Autodesk Inventor part; units mm, degrees
ref_plane "YZ Plane" through (0, 0, 0) normal (1, 0, 0) x (0, 1, 0)
ref_plane "XZ Plane" through (0, 0, 0) normal (0, 1, 0) x (-1, 0, 0)
ref_plane "XY Plane" through (0, 0, 0) normal (0, 0, 1) x (1, 0, 0)
sketch "Sketch1" plane through (0, 0, 0) normal (0, 0, 1) x (1, 0, 0)
  circle A0 centre (0, 0) radius 3
  circle A1 centre (0, 0) radius 6
  dimension "d0" = 6
  dimension "d1" = 12
extrude "Extrusion1" add sketch "Sketch1" against normal blind 3
sketch "Sketch2" plane through (0, 0, -3) normal (0, 0, -1) x (-1, 0, 0)
  circle A0 centre (0, 0) radius 7
  circle A1 centre (0, 0) radius 3
  dimension "d4" = 14
extrude "Extrusion2" add sketch "Sketch2" along normal blind 1
properties part number "Φ6-12a" material "Steel AISI 1006 85 HR"
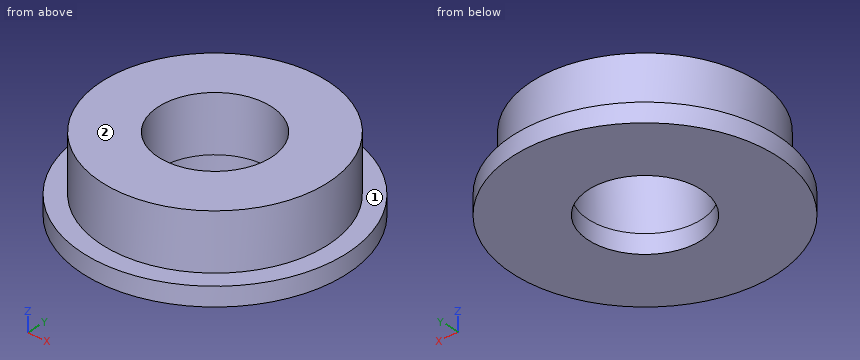
The listing builds one solid part. Answer for the finished solid, in the listing's coordinates (mm). Face numbers are marked on the shaded views. A direction names the side the tool comes from. Coordinates: 2 decimals unless noted, no trailing zeros. Loops run counter-clockwise (first coordinate to the right, second up) from the corner with the lowest first, then second, coordinate; pieces in that order, holes last. Notation, with made-up numbers: M -5,76.25 L -1,76.25 A28 cw -1,101.25 Z; hole C -10,2.25 d5. An arc over 180 degrees is marked long. Answer as a JSON object with one key per item and string values. Group by question number.
Item 1: Section D-D (z = -1.25) is taken. Write down the section's boundary in (x, y), and give its area (3 significant figures).
Item 2: Which of the six approach directions +Z, -Z, +X, -X, +Y, -Y give full straight-line access (tool end or side, diameter ignored) to the marked faces 1 and 2?
Item 3: Section A-A (x = 0) is taken. Write down the section's boundary in (y, z).
Item 4: Section C-C (x = 4.5) is taken. Write down the section's boundary in (y, z).
Item 5: Each of these flat-tipped pins is pushed along its axis until it touches: P1, Ø1, axis at x = -1, z = -2, coming from the -Y side; P2, Ø1, axis at x = -4.5, z = -0.5, coming from the +Y side; P3, Ø5.5, axis at x = 0, y = 0, coming from the -Z side. Where does it stop, or does it pass through?
Item 6: Consider L1, parallel to Y at x = 0, z = -0.6; L2, parallel to Y at x = 0, z = -3.4; L3, parallel to X at y = 2, z = -1.9. Determine where each line is inside the solid, lowest interval first.
Solved:
{
 "1": {"outline": "C 0,0 d12; hole C 0,0 d6", "area": "84.8 mm2"},
 "2": {"face 1": "+Z", "face 2": "+Z, +X, -X, +Y, -Y"},
 "3": {"outline": "M -7,-4 L -3,-4 L -3,0 L -6,0 L -6,-3 L -7,-3 Z; M 3,-4 L 7,-4 L 7,-3 L 6,-3 L 6,0 L 3,0 Z"},
 "4": {"outline": "M -5.36,-4 L 5.36,-4 L 5.36,-3 L 3.97,-3 L 3.97,0 L -3.97,0 L -3.97,-3 L -5.36,-3 Z"},
 "5": {"P1": "stops at y = -5.98", "P2": "stops at y = 4.47", "P3": "passes through"},
 "6": {"L1": "y = -6 to -3, 3 to 6", "L2": "y = -7 to -3, 3 to 7", "L3": "x = -5.66 to -2.24, 2.24 to 5.66"}
}
